from build123d import *

# Parameters (mm, degrees)
EXTRUDE_1_DEPTH              = 6
FILLET_2_R                   = 0.7
HOLE_WIZARD_M2_1_D           = 2.2
HOLE_WIZARD_M2_1_CBORE_D     = 4.6
HOLE_WIZARD_M2_1_CBORE_DEPTH = 3


with BuildPart() as part:
    # 草图1 → 凸台-拉伸1 (new body)
    with BuildSketch(Plane(origin=(0, 0, 0), x_dir=(1, 0, 0), z_dir=(0, 1, 0))):
        Polygon((-60, 40), (10, 40), (10, 25), (40, 25), (40, 15), (10, 15), (10, -30), (40, -30), (40, -40), (-60, -40), align=None)
    extrude(amount=EXTRUDE_1_DEPTH)

    # 圆角2
    fillet_2_edges = [part.edges().sort_by_distance(p)[0] for p in [
        (-25, 0, -40),
        (10, 0, -32.5),
        (25, 0, -25),
        (40, 0, -20),
        (25, 0, -15),
        (10, 0, 7.5),
        (25, 0, 30),
        (40, 6, 35),
        (40, 0, 35),
        (-10, 0, 40),
        (-60, 0, 0),
        (25, 6, 30),
        (-60, 3, -40),
        (10, 3, -40),
        (10, 3, -25),
        (40, 3, -25),
        (40, 3, -15),
        (10, 3, -15),
        (10, 3, 30),
        (40, 3, 30),
        (40, 3, 40),
        (-60, 3, 40),
        (10, 6, 7.5),
        (25, 6, -15),
        (40, 6, -20),
        (25, 6, -25),
        (10, 6, -32.5),
        (-25, 6, -40),
        (-60, 6, 0),
        (-10, 6, 40),
    ]]
    fillet(fillet_2_edges, radius=FILLET_2_R)

    # M2 六角头机械螺钉的柱形沉头孔1 (through all)
    with Locations(Plane(origin=(0, 6, 0), x_dir=(1, 0, 0), z_dir=(0, 1, 0))):
        with Locations((-20, 5), (-10, 5), (-10, -5), (-20, -5)):
            CounterBoreHole(HOLE_WIZARD_M2_1_D / 2, HOLE_WIZARD_M2_1_CBORE_D / 2, HOLE_WIZARD_M2_1_CBORE_DEPTH)


solid = part.part
Work out the finished part from the listing and answer in its coordinate system (mm). A direction names the side the tool comes from. Give positions to 0.01 mm unless a question says otherwise; leave off trailing zeros. Write each loop counter-clockwise with the first axis right and the second up, starting at its lowest first coordinate (ties: lowest second). Pieces come first, ordered by that corner, then holes. Notation, with made-up numbers: (22, 7) - (58, 7) arc R28 cw to (58, 28) - close; hole circle Ø4 at (46, 59.5). An arc over 180 degrees is marked (long way). One line per item, written item: value. Start each with the question number.
1. Find section D-D (x = -10). Write down the section's boundary in (y, z).
2. Find section B-B (x = 28). Write down the section's boundary in (y, z).
3. Consider probe 1 along X at (y, z) = (1.9, -5); probe 2 along Z at (x, y) = (-10, 1.3); probe 3 along Z at (x, y) = (-10, 5.2). Determine where each line is inside the solid, lowest interval first.
4. For faces 4 (the flat face through (-11, 3, -4)), 5 (the flat face through (-20, 6, -1)), 6 (the flat face through (10, 3, -33)), determine the directions among +Z, -Z, +X, -X, +Y, -Y from which every point of the face is accessible in a straight line to the end or side of a thin tool.
5. Find section A-A (z = -5). Write down the section's boundary in (x, y), then the cut area to 3 significant figures.
6. For a pull along X with two mould halves and no side action, classify faces 1 (the flat face through (-60, 3, 1)), 2 (the cylindrical face through (-11.825, 4.521, 6.4)), 3 (the flat face through (25, 3, 30)) as +X half, -X half, draft (parallel to the pull), parting line (faces both ways), or undercut.
7. Find section C-C (y = 1.75). Write down the section's boundary in (x, z), then the cut area to 3 significant figures.
8. Given pin 1 (1.5 mm diameter, centred on x = 27, y = 2.5, fed in from -Z); pin 2 (4 mm diameter, centred on x = -20, z = -5, fed in from -Y); pin 3 (3.5 mm diameter, centred on y = 2.5, z = -35, fed in from +X); pin 4 (1.4 mm diameter, centred on x = -9, z = -5.5, fed in from +Y), each flat-ended and moving along its own axis, determine where each tip first touches the part or whether it passes through.
Geometry results:
1. outline: (0, -39.3) arc R0.7 ccw to (0.7, -40) - (5.3, -40) arc R0.7 ccw to (6, -39.3) - (6, -7.3) - (3, -7.3) - (3, -6.1) - (0, -6.1) - close; (0, -3.9) - (3, -3.9) - (3, -2.7) - (6, -2.7) - (6, 2.7) - (3, 2.7) - (3, 3.9) - (0, 3.9) - close; (0, 6.1) - (3, 6.1) - (3, 7.3) - (6, 7.3) - (6, 39.3) arc R0.7 ccw to (5.3, 40) - (0.7, 40) arc R0.7 ccw to (0, 39.3) - close
2. outline: (0, -24.3) arc R0.7 ccw to (0.7, -25) - (5.3, -25) arc R0.7 ccw to (6, -24.3) - (6, -15.7) arc R0.7 ccw to (5.3, -15) - (0.7, -15) arc R0.7 ccw to (0, -15.7) - close; (0, 30.7) arc R0.7 ccw to (0.7, 30) - (5.3, 30) arc R0.7 ccw to (6, 30.7) - (6, 39.3) arc R0.7 ccw to (5.3, 40) - (0.7, 40) arc R0.7 ccw to (0, 39.3) - close
3. probe 1: -60 to -21.1, -18.9 to -11.1, -8.9 to 10
3. probe 2: -40 to -6.1, -3.9 to 3.9, 6.1 to 40
3. probe 3: -40 to -7.3, -2.7 to 2.7, 7.3 to 40
4. face 4: +Y
4. face 5: +Z, -Z, +X, -X, +Y
4. face 6: -Z, +X, +Y, -Y
5. outline: (-60, 0.7) arc R0.7 ccw to (-59.3, 0) - (-21.1, 0) - (-21.1, 3) - (-22.3, 3) - (-22.3, 6) - (-59.3, 6) arc R0.7 ccw to (-60, 5.3) - close; (-18.9, 0) - (-11.1, 0) - (-11.1, 3) - (-12.3, 3) - (-12.3, 6) - (-17.7, 6) - (-17.7, 3) - (-18.9, 3) - close; (-8.9, 0) - (9.3, 0) arc R0.7 ccw to (10, 0.7) - (10, 5.3) arc R0.7 ccw to (9.3, 6) - (-7.7, 6) - (-7.7, 3) - (-8.9, 3) - close
5. area: 379 mm2
6. face 1: -X half
6. face 2: undercut
6. face 3: draft
7. outline: (-60, -39.3) arc R0.7 ccw to (-59.3, -40) - (9.3, -40) arc R0.7 ccw to (10, -39.3) - (10, -25.7) arc R0.7 cw to (10.7, -25) - (39.3, -25) arc R0.7 ccw to (40, -24.3) - (40, -15.7) arc R0.7 ccw to (39.3, -15) - (10.7, -15) arc R0.7 cw to (10, -14.3) - (10, 29.3) arc R0.7 cw to (10.7, 30) - (39.3, 30) arc R0.7 ccw to (40, 30.7) - (40, 39.3) arc R0.7 ccw to (39.3, 40) - (-59.3, 40) arc R0.7 ccw to (-60, 39.3) - close; hole circle Ø2.2 at (-20, -5); hole circle Ø2.2 at (-20, 5); hole circle Ø2.2 at (-10, -5); hole circle Ø2.2 at (-10, 5)
7. area: 6,180 mm2
8. pin 1: z = -25
8. pin 2: y = 0
8. pin 3: x = 10
8. pin 4: y = 3
